```python
from build123d import *

# Parameters (mm, degrees)
F1_DEPTH = 19.05
F2_W     = 279.4
F2_H     = 19.05
F2_W_2   = 241.3
F2_W_3   = 19.05
F2_H_2   = 76.2
F3_DEPTH = 406.4
F5_DEPTH = 19.05
F7_DEPTH = 19.05


with BuildPart() as f1:
    # F0 (on Right) → F1 (new body)
    with BuildSketch(Plane.YZ):
        Polygon((76.2, 355.6), (0, 0), (304.8, 0), (304.8, 355.6), align=None)
    extrude(amount=F1_DEPTH)

    # F2 (on face) → F3 (join)
    with BuildSketch(Plane(origin=(0, 0, 0), x_dir=(0, -1, 0), z_dir=(-1, 0, 0))):
        with Locations((-165.1, 34.925)):
            Rectangle(F2_W, F2_H)
        with Locations((-184.15, 200.025)):
            Rectangle(F2_W_2, F2_H)
        with Locations((-295.275, 317.5)):
            Rectangle(F2_W_3, F2_H_2)
    extrude(amount=F3_DEPTH)

    # F4 (on face) → F5 (join)
    with BuildSketch(Plane(origin=(-406.4, 0, 0), x_dir=(0, -1, 0), z_dir=(-1, 0, 0))):
        Polygon((-304.8, 0), (0, 0), (-76.2, 355.6), (-304.8, 355.6), align=None)
    extrude(amount=F5_DEPTH)

    # F6 (on face) → F7 (join)
    with BuildSketch(Plane.XY.offset(355.6)):
        with BuildLine():
            Line((38.1, 69.85), (38.1, 304.8))
            Line((38.1, 304.8), (-444.5, 304.8))
            Line((-444.5, 304.8), (-444.5, 63.5))
            ThreePointArc((-444.5, 63.5), (-440.780256, 54.519744), (-431.8, 50.8))
            Line((-431.8, 50.8), (19.05, 50.8))
            ThreePointArc((19.05, 50.8), (32.520384, 56.379616), (38.1, 69.85))
        make_face()
    extrude(amount=F7_DEPTH)


solid = f1.part
```
Here's how the part is built. I have some questions about the finished solid (model axes, mm). A direction names the side the tool comes from. Give positions to 0.01 mm unless a question says otherwise; leave off trailing zeros. Order: outer loops, then holes, each group sorted by start corner. A loop starts at its lowest first (then second) coordinate and runs counter-clockwise, first axis right, second up. Notation, with made-up numbers: (54, 51) -> (85, 51) arc R19 cw to (85, 63) -> close; hole circle Ø4 at (8.25, -32). An arc over 180 degrees is marked (long way). Use CSV: the item, a comma, the result in double quotes. Start each with the question number.
Item 1: Suppose I cut it at C-C (y = 184). List the corners of the cut face in (x, z) for me.
Item 2: Suppose I cut it at B-B (z = 98). List the corners of the cut face in (x, y) for me.
Item 3: I'm going to push flat-ended pins straight in: P1, Ø21, axis at x = -156, z = 199, coming from the -Y side; P2, Ø2, axis at y = 44.5, z = 134.5, coming from the -X side; P3, Ø10, axis at x = -183, y = 202.5, coming from the -Z side. Where does each tip first touch, or does it pass through?
Item 4: Suppose I cut it at A-A (x = -322). List the corners of the cut face in (y, z) for me, and give its area (3 significant figures).
Item 5: If I drill on probe 1 along Z at (x, y) = (-187, 99.5); probe 2 along X at (y, z) = (257.5, 325); probe 3 along Z at (x, y) = (-252, 57.5), over which ranges is the centre line in solid material (lowest first)? Write a range as [from, to].
Item 6: Suppose I cut it at D-D (y = 45). List the corners of the cut face in (x, z) for me, and give its area (3 significant figures).
Item 7: Thinking about a two-plate mould opening in Z: for faces 6 (the flat face through (-415.792, 37.567, 175.311)), 7 (the flat face through (-210, 50.8, 365)), 8 (the flat face through (-207, 180, 374.65)), which applies, pulls with the +Z half, pulls with the -Z half, needs draft (parallel to the pull), parting line crosses it, or undercut?
Item 8: On a 3-axis mill with a long thin cutter (end or side, diameter ignored), from which of +Z, -Z, +X, -X, +Y, -Y can I reach the whole of each face in a straight line? I mean faces 1 (the flat face through (-200, 63.5, 200)), 2 (the flat face through (-200, 186, 190.5)), 3 (the flat face through (-200, 25.4, 35)), 4 (the flat face through (19.05, 184, 180)), 5 (the flat face through (-200, 167, 25.4)). Say none if no direction works.
Answer block:
1,outline,"(-444.5, 355.6) -> (-425.45, 355.6) -> (-425.45, 0) -> (-406.4, 0) -> (-406.4, 25.4) -> (0, 25.4) -> (0, 0) -> (19.05, 0) -> (19.05, 355.6) -> (38.1, 355.6) -> (38.1, 374.65) -> (-444.5, 374.65) -> close; hole (-406.4, 44.45) -> (0, 44.45) -> (0, 190.5) -> (-406.4, 190.5) -> close; hole (-406.4, 209.55) -> (0, 209.55) -> (0, 355.6) -> (-406.4, 355.6) -> close"
2,outline,"(-425.45, 21) -> (-406.4, 21) -> (-406.4, 304.8) -> (-425.45, 304.8) -> close; (0, 21) -> (19.05, 21) -> (19.05, 304.8) -> (0, 304.8) -> close"
3,P1,"stops at y = 63.5"
3,P2,"stops at x = -425.45"
3,P3,"stops at z = 25.4"
4,outline,"(25.4, 25.4) -> (304.8, 25.4) -> (304.8, 44.45) -> (25.4, 44.45) -> close; (50.8, 355.6) -> (285.75, 355.6) -> (285.75, 279.4) -> (304.8, 279.4) -> (304.8, 374.65) -> (50.8, 374.65) -> close; (63.5, 190.5) -> (304.8, 190.5) -> (304.8, 209.55) -> (63.5, 209.55) -> close"
4,area,"16,200 mm^2"
5,probe 1,"z = [25.4, 44.45], [190.5, 209.55], [355.6, 374.65]"
5,probe 2,"x = [-425.45, -406.4], [0, 19.05]"
5,probe 3,"z = [25.4, 44.45], [355.6, 374.65]"
6,outline,"(-425.45, 0) -> (-406.4, 0) -> (-406.4, 25.4) -> (0, 25.4) -> (0, 0) -> (19.05, 0) -> (19.05, 210) -> (0, 210) -> (0, 44.45) -> (-406.4, 44.45) -> (-406.4, 210) -> (-425.45, 210) -> close"
6,area,"15,700 mm^2"
7,face 6,"undercut"
7,face 7,"needs draft"
7,face 8,"pulls with the +Z half"
8,face 1,"-Y"
8,face 2,"+Y, -Y"
8,face 3,"+Z, -Z, -Y"
8,face 4,"-Z, +X, +Y, -Y"
8,face 5,"-Z, +Y, -Y"
